For this review, take the finished solid that the model builds, in its own axes (mm). A direction names the side the tool comes from. Round coordinates to 2 decimals unless told otherwise and drop trailing zeros. Order: outer loops, then holes, each group sorted by start corner. A loop starts at its lowest first (then second) coordinate and runs counter-clockwise, first axis right, second up. Notation, with made-up numbers: M 17.5,-1.75 L 39.5,-1.75 A20 cw 39.5,7.25 Z; hole C 65.25,78 d8. An arc over 180 degrees is marked long. Use a Markdown table: item, result.
Autodesk Inventor part; units mm, degrees
ref_plane "Start Plane" through (0, 0, 0) normal (0, 0, 1) x (1, 0, 0)
ref_plane "End Plane" through (0, 0, 520) normal (0, 0, 1) x (1, 0, 0)
ref_plane "YZ Plane" through (0, 0, 0) normal (1, 0, 0) x (0, 1, 0)
ref_plane "Start Plane" through (0, 0, 0) normal (0, 0, 1) x (1, 0, 0)
ref_plane "End Plane" through (0, 0, 520) normal (0, 0, 1) x (1, 0, 0)
sketch "Sketch" plane through (0, 0, 0) normal (0, 0, 1) x (1, 0, 0)
  line L0 (-20, -16) -> (-20, 16)
  line L1 (-16, 20) -> (16, 20)
  line L2 (20, 16) -> (20, -16)
  line L3 (16, -20) -> (-16, -20)
  arc A0 (-20, -16) -> (-16, -20) centre (-16, -16) ccw
  arc A1 (20, 16) -> (16, 20) centre (16, 16) ccw
  arc A2 (-16, 20) -> (-20, 16) centre (-16, 16) ccw
  arc A3 (16, -20) -> (20, -16) centre (16, -16) ccw
  arc A4 (-16, 18) -> (-18, 16) centre (-16, 16) ccw
  line L4 (-16, 18) -> (16, 18)
  arc A5 (18, 16) -> (16, 18) centre (16, 16) ccw
  line L5 (18, 16) -> (18, -16)
  arc A6 (16, -18) -> (18, -16) centre (16, -16) ccw
  line L6 (16, -18) -> (-16, -18)
  arc A7 (-18, -16) -> (-16, -18) centre (-16, -16) ccw
  line L7 (-18, -16) -> (-18, 16)
  line L8 (0, 29.1598) -> (0, -29.1598) construction
  line L9 (-29.1598, 0) -> (29.1598, 0) construction
  dimension "d7" = 4
  dimension "d9" = 40
  dimension "d11" = 40
  dimension "d12" = 2
  dimension "d15" = 20
  dimension "d16" = 20
extrude "Body" add sketch "Sketch" along normal up to surface (520 mm away) from surface at 0
sketch "Sketch3" plane through (0, 0, 0) normal (0, 0, 1) x (1, 0, 0)
  line L0 (0, 0) -> (10, 0)
ref_plane "Work Plane3" through (0, 0, 0) normal (0, -1, 0) x (1, 0, 0)
sketch "Sketch4" plane through (0, 0, 0) normal (0, -1, 0) x (1, 0, 0)
  line L0 (-2, 0) -> (12, 0)
  line L1 (-2, 520) -> (12, 520)
  dimension "d18" = 520
equation "\"d7\" = G_IR"
equation "\"d9\" = G_W"
equation "\"d11\" = G_H"
equation "\"d12\" = G_T"
equation "\"d15\" = 0.5 * d9"
equation "\"d16\" = 0.5 * d11"
equation "\"d3\" = G_L"
equation "\"G_W\" = 40"
equation "\"G_H\" = 40"
equation "\"G_T\" = 2"
equation "\"G_IR\" = 4"
equation "\"G_L\" = d18"
equation "\"G_OFFSET_START\" = 0"
equation "\"G_OFFSET_END\" = -6"
equation "\"B_L\" = 526"
properties part number "ISO 10799-2 - 40x40x2 - 520" material "Stainless Steel"
Q1. Wall thickness on line 1 along X through (y, z) = (-14, 434.5); line 2 along X through (y, z) = (17, 308): over which ranges is each line inside the solid? List them lowest first. Write a range as [from, to].
Determined:
| item | result |
|---|---|
| line 1 | x = [-20, -18], [18, 20] |
| line 2 | x = [-19.87, -17.73], [17.73, 19.87] |
Q2. Add section C-C (z = 141). Write out the cut boundary in (x, y), then the cut area to 3 significant figures.
Determined:
| item | result |
|---|---|
| outline | M -20,-16 A4 ccw -16,-20 L 16,-20 A4 ccw 20,-16 L 20,16 A4 ccw 16,20 L -16,20 A4 ccw -20,16 Z; hole M -18,-16 A2 ccw -16,-18 L 16,-18 A2 ccw 18,-16 L 18,16 A2 ccw 16,18 L -16,18 A2 ccw -18,16 Z |
| area | 294 mm^2 |
Q3. Machinability: for faces 4 (the flat face through (-2, -19, 0)), 5 (the flat face through (18, 0, 256)), which of the approach directions +Z, -Z, +X, -X, +Y, -Y give a long, thin tool a straight path to every point of the face, cutting with its end or side? Answer none if there is none.
Determined:
| item | result |
|---|---|
| face 4 | -Z, +X, -X, +Y, -Y |
| face 5 | +Z, -Z |
Q4. Add section A-A (x = -11). Write out the cut boundary in (y, z), then the cut area to 3 significant figures.
Determined:
| item | result |
|---|---|
| outline | M -20,0 L -18,0 L -18,520 L -20,520 Z; M 18,0 L 20,0 L 20,520 L 18,520 Z |
| area | 2,080 mm^2 |
Q5. Draft analysis for pull direction Y (two halves, no side actions). For faces 1 (the flat face through (-18, 0, 256)), 2 (the flat face through (-20, 0, 256)), 3 (the flat face through (0, -20, 256)), state which applies: pulls with the +Y half, pulls with the -Y half, needs draft (parallel to the pull), parting line crosses it, or undercut.
Determined:
| item | result |
|---|---|
| face 1 | undercut |
| face 2 | needs draft |
| face 3 | pulls with the -Y half |
